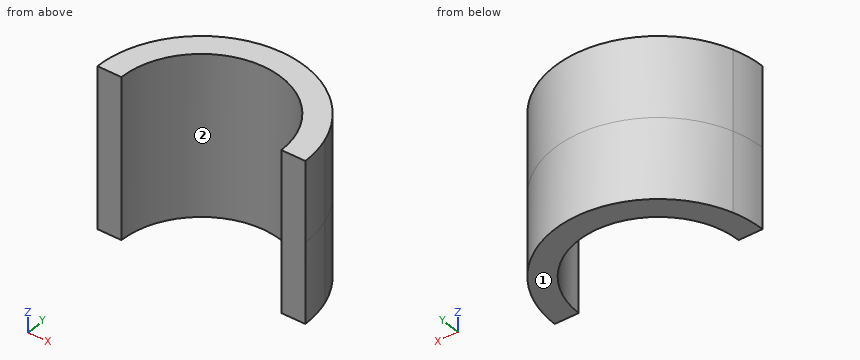
from build123d import *

# Parameters (mm, degrees)
BOSS_EXTRUDE1_DEPTH = 31.75


with BuildPart() as part:
    # Sketch1 → Boss-Extrude1 (new body, symmetric)
    with BuildSketch(Plane.XY):
        with BuildLine():
            ThreePointArc((57.15, 0), (88.9, 31.75), (120.65, 0))
            Line((120.65, 0), (130.175, 0))
            ThreePointArc((130.175, 0), (129.671322086, 6.428446187), (128.172581084, 12.7))
            ThreePointArc((128.172581084, 12.7), (88.9, 41.275), (49.627418916, 12.7))
            ThreePointArc((49.627418916, 12.7), (48.128677914, 6.428446187), (47.625, 0))
            Line((47.625, 0), (57.15, 0))
        make_face()
    extrude(amount=BOSS_EXTRUDE1_DEPTH, both=True)


solid = part.part
Here's how the part is built. I have some questions about the finished solid (model axes, mm). Face numbers are marked on the shaded views. Give positions to 0.01 mm unless a question says otherwise; leave off trailing zeros. Write each loop counter-clockwise with the first axis right and the second up, starting at its lowest first coordinate (ties: lowest second). Pieces come first, ordered by that corner, then holes. Notation, with made-up numbers: (5, -12) -> (26, -12) arc R13 cw to (26, 6) -> close; hole circle Ø1 at (-27.75, -22). An arc over 180 degrees is marked (long way). Use one line per item in the form item = value. Start each with the question number.
1. Imagine slicing it at A-A on y = 8. List the corners of the cut face in (x, z) for me, plus the area to 3 significant figures.
2. Will these pins go through, and if not, where does the flat tip stop? pin 1 Ø10 at (x, z) = (120.5, 9.5) entering from +Y; pin 2 Ø6 at (y, z) = (20.5, 23) entering from -X; pin 3 Ø8 at (y, z) = (5, 10.5) entering from +X.
3. Imagine slicing it at C-C on y = 21.5. List the corners of the cut face in (x, z) for me.
4. If I drill on L1, parallel to X at y = 8.5, z = 20.5; L2, parallel to X at y = 22.5, z = -24.5; L3, parallel to Y at x = 117, z = -6, over which ranges is the centre line in solid material (lowest first)?
5. Imagine slicing it at D-D on x = 88.9. List the corners of the cut face in (y, z) for me (3 decimals).
6. Imagine slicing it at B-B on z = -12. List the corners of the cut face in (x, y) for me (3 decimals), plus the area to 3 significant figures.
7. Thinking about a two-plate mould opening in X: for the marked faces 1 and 2, which applies, +X half, -X half, draft (parallel to the pull), parting line (faces both ways), or undercut?
Entries:
q1.outline = (48.41, -31.75) -> (58.17, -31.75) -> (58.17, 31.75) -> (48.41, 31.75) -> close; (119.63, -31.75) -> (129.39, -31.75) -> (129.39, 31.75) -> (119.63, 31.75) -> close
q1.area = 1,240 mm²
q2.pin_1 = 31.56
q2.pin_2 = 51.52
q2.pin_3 = 130.16
q3.outline = (53.67, -31.75) -> (65.54, -31.75) -> (65.54, 31.75) -> (53.67, 31.75) -> close; (112.26, -31.75) -> (124.13, -31.75) -> (124.13, 31.75) -> (112.26, 31.75) -> close
q4.L1 = 48.51 to 58.31, 119.49 to 129.29
q4.L2 = 54.3 to 66.5, 111.3 to 123.5
q4.L3 = 14.78 to 30.23
q5.outline = (31.75, -31.75) -> (41.275, -31.75) -> (41.275, 31.75) -> (31.75, 31.75) -> close
q6.outline = (47.625, 0) -> (57.15, 0) arc R31.75 cw to (120.65, 0) -> (130.175, 0) arc R41.275 ccw to start
q6.area = 1,090 mm²
q7.face_1 = draft
q7.face_2 = undercut
